Read the model definition and answer for the solid it produces. Units are mm, in the model's axes. Coordinates: 2 decimals unless noted, no trailing zeros. Write each loop counter-clockwise with the first axis right and the second up, starting at its lowest first coordinate (ties: lowest second). Pieces come first, ordered by that corner, then holes.
(1) A straight line is drawn through the part: line 1 along Y through (x, z) = (21.5, 23). Find the intervals that lie inside material, in ascending order.
(2) The part is cut by section B-B, the plane z = 2. Determine the outline of the cut face in (x, y).
(3) Given pin 1 (3 mm diameter, centred on x = 6, z = 24.5, fed in from +Y), flat-ended and moving along its own axis, determine where the tip first touches the part or whether it passes through.
(4) The part is cut by section A-A, the plane x = 15.5. Determine the outline of the cut face in (y, z), and give its area (3 significant figures).
Autodesk Inventor part; units mm, degrees
ref_plane "MidPlane" through (0, 2.3, -2.4) normal (0, 0, 1) x (1, 0, 0)
ref_plane "YZ Plane" through (0, 0, 0) normal (1, 0, 0) x (0, 1, 0)
ref_plane "XZ Plane" through (0, 0, 0) normal (0, 1, 0) x (-1, 0, 0)
sketch "Sketch1" plane through (0, 0, 0) normal (0, 1, 0) x (-1, 0, 0)
  line L0 (27.33, 41.47) -> (-27.33, 41.47)
  line L1 (-27.33, 41.47) -> (-27.33, -41.47)
  line L2 (-27.33, -41.47) -> (27.33, -41.47)
  line L3 (27.33, -41.47) -> (27.33, 41.47)
  line L4 (27.33, 41.47) -> (-27.33, -41.47) construction
  line L5 (-27.33, 41.47) -> (27.33, -41.47) construction
  point P0 (0, 0)
  dimension "d0" = 82.94
  dimension "d1" = 54.66
extrude "Extrusion1" add sketch "Sketch1" along normal blind 2.3
sketch "Sketch2" plane through (0, 2.3, 0) normal (0, 1, 0) x (1, 0, 0)
  line L0 (-24.98, 39.62) -> (24.98, 39.62)
  line L1 (24.98, 39.62) -> (24.98, -34.82)
  line L2 (24.98, -34.82) -> (-24.98, -34.82)
  line L3 (-24.98, -34.82) -> (-24.98, 39.62)
  line L4 (-24.98, 39.62) -> (24.98, -34.82) construction
  line L5 (24.98, 39.62) -> (-24.98, -34.82) construction
  line L6 (27.33, 41.47) -> (-27.33, 41.47)
  point P0 (0, 0)
  point P1 (0, 2.4)
  dimension "d4" = 74.44
  dimension "d5" = 49.96
  dimension "d6" = 1.85
extrude "Extrusion2" cut sketch "Sketch2" against normal blind 0.05
ref_plane "MidPlane" through (0, 2.3, -2.4) normal (0, 0, 1) x (1, 0, 0)
properties part number "Multi-Inno_3.5in_LCD"
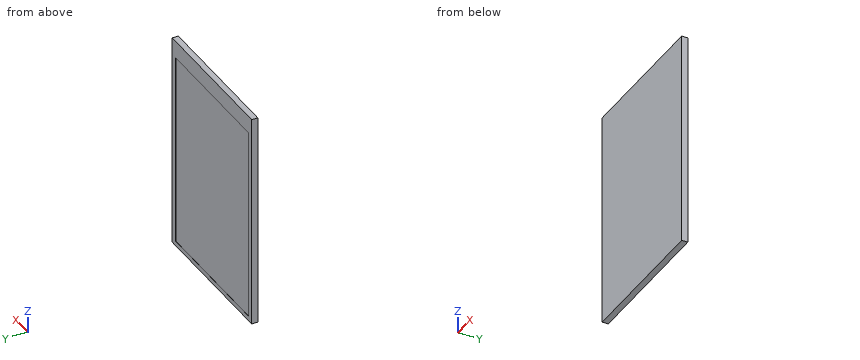
Computed:
1. line 1: y = 0 to 2.25
2. outline: (-27.33, 0) - (27.33, 0) - (27.33, 2.3) - (24.98, 2.3) - (24.98, 2.25) - (-24.98, 2.25) - (-24.98, 2.3) - (-27.33, 2.3) - close
3. pin 1: stops at y = 2.25
4. outline: (0, -41.47) - (2.3, -41.47) - (2.3, -39.62) - (2.25, -39.62) - (2.25, 34.82) - (2.3, 34.82) - (2.3, 41.47) - (0, 41.47) - close
4. area: 187 mm2
